Model file for the job. Use its own axes, mm. A direction names the side the tool comes from. Coordinates: 2 decimals unless noted, no trailing zeros. Write each loop counter-clockwise with the first axis right and the second up, starting at its lowest first coordinate (ties: lowest second). Pieces come first, ordered by that corner, then holes. Notation, with made-up numbers: (44, 14) -> (81, 14) arc R20 cw to (81, 30) -> close; hole circle Ø4 at (68, 48.5). An arc over 180 degrees is marked (long way). Answer as a JSON object with one key per item and string values. Group by question number.
from build123d import *

# Parameters (mm, degrees)
SKETCH_W        = 100
SKETCH_H        = 140
PAD_DEPTH       = 21
SKETCH001_W     = 90
SKETCH001_H     = 135
POCKET_DEPTH    = 15
SKETCH003_R     = 3
POCKET001_DEPTH = 2
SKETCH004_R     = 1.6
POCKET002_DEPTH = 350.647794
SKETCH005_W     = 5
SKETCH005_H     = 50
POCKET003_DEPTH = 21.001
SKETCH006_W     = 30
SKETCH006_H     = 5
POCKET004_DEPTH = 21.001
FILLET_R        = 5
POCKET005_DEPTH = 5
FILLET001_R     = 15
SKETCH008_R     = 5
PAD001_DEPTH    = 5
FILLET002_R     = 4.9
SKETCH009_R     = 5
PAD002_DEPTH    = 5
FILLET003_R     = 4.9


with BuildPart() as part:
    # Sketch → Pad (new body)
    with BuildSketch(Plane.XY):
        Rectangle(SKETCH_W, SKETCH_H)
    extrude(amount=PAD_DEPTH)

    # Sketch001 → Pocket (cut)
    with BuildSketch(Plane.XY.offset(21)):
        with Locations((0, 2.5)):
            Rectangle(SKETCH001_W, SKETCH001_H)
    extrude(amount=-POCKET_DEPTH, mode=Mode.SUBTRACT)

    # Sketch003 → Pocket001 (cut)
    with BuildSketch(Plane.XY.offset(6)):
        with Locations((-15, -25)):
            Circle(SKETCH003_R)
    pocket001 = extrude(amount=-POCKET001_DEPTH, mode=Mode.SUBTRACT)

    # Sketch004 → Pocket002 (cut, through all)
    with BuildSketch(Plane.XY.offset(4)):
        with Locations((-15, -25)):
            Circle(SKETCH004_R)
    pocket002 = extrude(amount=-POCKET002_DEPTH, mode=Mode.SUBTRACT)

    # Mirrored: Pocket002, Pocket001 across Sketch004 V_Axis
    add(pocket002.mirror(Plane(origin=(0, 0, 4), x_dir=(0, 0, 1), z_dir=(1, 0, 0))), mode=Mode.SUBTRACT)
    add(pocket001.mirror(Plane(origin=(0, 0, 4), x_dir=(0, 0, 1), z_dir=(1, 0, 0))), mode=Mode.SUBTRACT)

    # Sketch005 → Pocket003 (cut, through all)
    with BuildSketch(Plane.XY.offset(21)):
        with Locations((47.5, 30)):
            Rectangle(SKETCH005_W, SKETCH005_H)
    extrude(amount=-POCKET003_DEPTH, mode=Mode.SUBTRACT)

    # Sketch006 → Pocket004 (cut, through all)
    with BuildSketch(Plane.XY.offset(21)):
        with Locations((0, -67.5)):
            Rectangle(SKETCH006_W, SKETCH006_H)
    extrude(amount=-POCKET004_DEPTH, mode=Mode.SUBTRACT)

    # Fillet
    fillet_edges = [part.edges().sort_by_distance(p)[0] for p in [
        (-50, -70, 10.5),
        (50, -70, 10.5),
    ]]
    fillet(fillet_edges, radius=FILLET_R)

    # Sketch007 → Pocket005 (cut)
    with BuildSketch(Plane(origin=(0, 0, 0), x_dir=(1, 0, 0), z_dir=(0, 0, -1))):
        with BuildLine():
            Line((9, 30), (9, 21.392622))
            ThreePointArc((-9, 21.392622), (0, -29), (9, 21.392622))
            Line((-9, 21.392622), (-9, 30))
            Line((-17, 30), (-9, 30))
            Line((-17, 63), (-17, 30))
            Line((-4.261222, 63), (-17, 63))
            Line((-4.261222, 63), (-4.261222, 65))
            Line((-4.261222, 65), (4.261222, 65))
            Line((4.261222, 65), (4.261222, 63))
            Line((17, 63), (4.261222, 63))
            Line((17, 30), (17, 63))
            Line((9, 30), (17, 30))
        make_face()
    extrude(amount=-POCKET005_DEPTH, mode=Mode.SUBTRACT)

    # Fillet001
    fillet001_edges = [part.edges().sort_by_distance(p)[0] for p in [
        (-15, -67.5, 21),
        (15, -67.5, 21),
    ]]
    fillet(fillet001_edges, radius=FILLET001_R)

    # Sketch008 → Pad001 (new body)
    with BuildSketch(Plane.XY.offset(6)):
        with Locations((-39.8, 64.8)):
            Circle(SKETCH008_R)
    pad001 = extrude(amount=PAD001_DEPTH)

    # Mirrored001: Pad001 across Sketch008 V_Axis
    add(pad001.mirror(Plane(origin=(0, 0, 6), x_dir=(0, 0, 1), z_dir=(1, 0, 0))))

    # Fillet002
    fillet002_edges = [part.edges().sort_by_distance(p)[0] for p in [
        (-44.8, 64.8, 11),
        (44.8, 64.8, 11),
    ]]
    fillet(fillet002_edges, radius=FILLET002_R)

    # Sketch009 → Pad002 (new body)
    with BuildSketch(Plane.XY.offset(6)):
        with Locations((-39.8, -50)):
            Circle(SKETCH009_R)
    pad002 = extrude(amount=PAD002_DEPTH)

    # Mirrored002: Pad002 across Sketch009 V_Axis
    add(pad002.mirror(Plane(origin=(0, 0, 6), x_dir=(0, 0, 1), z_dir=(1, 0, 0))))

    # Fillet003
    fillet003_edges = [part.edges().sort_by_distance(p)[0] for p in [
        (-44.8, -50, 11),
        (44.8, -50, 11),
    ]]
    fillet(fillet003_edges, radius=FILLET003_R)


solid = part.part
(1) Cut at C-C on y = 3. List the corners of the cut face in (x, z).
(2) Cut at D-D on x = 0. List the corners of the cut face in (y, z), plus the area to 3 significant figures.
(3) Wall check: probe 1 along X at (y, z) = (-6.5, 9.25); probe 2 along X at (y, z) = (3, 2.95); probe 3 along Y at (x, z) = (-11, 4.5). Give the ranges that are in metal, low to high.
(4) Pin check, flat tips, straight feed: pin 1 (8 mm diameter, centred on x = -19.5, y = -28.5, fed in from +Z); pin 2 (2.5 mm diameter, centred on x = 15, y = -25, fed in from -Z); pin 3 (7.5 mm diameter, centred on x = -28, z = 14, fed in from +Y); pin 4 (4 mm diameter, centred on x = 13.5, z = 3.5, fed in from -Y). Stop position of each tip, or through.
(5) Pull direction Y, two halves, no side cores. Call faces 1 (the face through (49, -68, 11)), 2 (the face through (45, 30, 3)), 3 (the face through (-11.8, 70, 5.7)): released by +Y, released by -Y, zero draft, split by the parting line, or undercut.
(6) Cut at B-B on y = -25. List the corners of the cut face in (x, z), plus the area to 3 significant figures.
(7) 3-axis set-ups, long thin cutter, end or side, ignore diameter. For faces 4 (the face through (19.28, -67.46, 16.49)), 5 (the face through (-45, 2, 14)), 6 (the face through (0, -19, 5)), 7 (the face through (-15, -68, 3)), 8 (the face through (18, -25, 5)): which of +Z, -Z, +X, -X, +Y, -Y reach the whole face in a straight line?
(8) Cut at A-A on z = 18. List the corners of the cut face in (x, y).
Results found:
{
 "1": {"outline": "(-50, 0) -> (-26, 0) -> (-26, 5) -> (26, 5) -> (26, 0) -> (50, 0) -> (50, 21) -> (45, 21) -> (45, 6) -> (-45, 6) -> (-45, 21) -> (-50, 21) -> close"},
 "2": {"outline": "(-65, 5) -> (29, 5) -> (29, 0) -> (70, 0) -> (70, 6) -> (-65, 6) -> close", "area": "340 mm²"},
 "3": {"probe 1": "x = -50 to -45, 45 to 50", "probe 2": "x = -50 to -26, 26 to 50", "probe 3": "y = -65 to -63, -30 to -20.56, 26.56 to 70"},
 "4": {"pin 1": "stops at z = 6", "pin 2": "passes through", "pin 3": "stops at y = -65", "pin 4": "stops at y = -70"},
 "5": {"face 1": "released by -Y", "face 2": "undercut", "face 3": "released by +Y"},
 "6": {"outline": "(-50, 0) -> (-16.6, 0) -> (-16.6, 4) -> (-18, 4) -> (-18, 6) -> (-45, 6) -> (-45, 21) -> (-50, 21) -> close; (-13.4, 0) -> (-9, 0) -> (-9, 5) -> (9, 5) -> (9, 0) -> (13.4, 0) -> (13.4, 4) -> (12, 4) -> (12, 6) -> (-12, 6) -> (-12, 4) -> (-13.4, 4) -> close; (16.6, 0) -> (50, 0) -> (50, 21) -> (45, 21) -> (45, 6) -> (18, 6) -> (18, 4) -> (16.6, 4) -> close", "area": "610 mm²"},
 "7": {"face 4": "+Z, +Y, -Y", "face 5": "+Z, +Y", "face 6": "-Z", "face 7": "+Z, -Z, -Y", "face 8": "+Z"},
 "8": {"outline": "(-50, -65) arc R5 ccw to (-45, -70) -> (-21, -70) -> (-21, -65) -> (-45, -65) -> (-45, 70) -> (-50, 70) -> close; (21, -70) -> (45, -70) arc R5 ccw to (50, -65) -> (50, 5) -> (45, 5) -> (45, -65) -> (21, -65) -> close; (45, 55) -> (50, 55) -> (50, 70) -> (45, 70) -> close"}
}
